Read the model definition and answer for the solid it produces. Units are mm, in the model's axes. Face numbers are marked on the shaded views. A direction names the side the tool comes from. Round coordinates to 2 decimals unless told otherwise and drop trailing zeros. Loops run counter-clockwise (first coordinate to the right, second up) from the corner with the lowest first, then second, coordinate; pieces in that order, holes last. Notation, with made-up numbers: M 27.5,43 L 48.5,43 A8 ccw 48.5,51 Z; hole C 25.5,-6.75 d4. An arc over 180 degrees is marked long. Write each question's results on one line, items separated by ' | '.
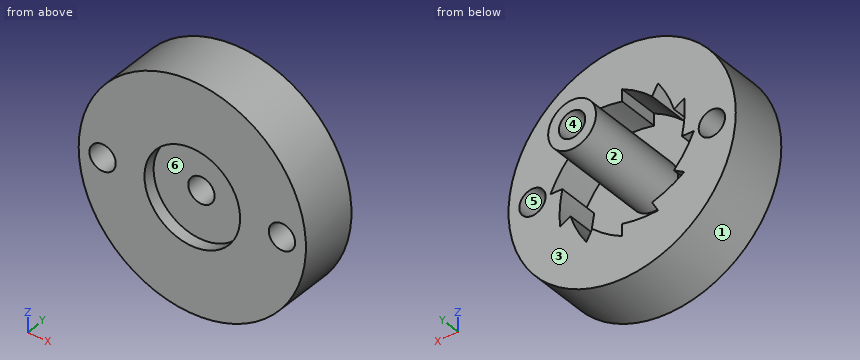
from build123d import *

# Parameters (mm, degrees)
SIDE_PROFILE_RATCHETING_PULLEY_MASTERMOD_W = 7.5
SIDE_PROFILE_RATCHETING_PULLEY_MASTERMOD_H = 5
RATCHETING_START                           = 1.5
RATCHETING_PULLEY_MASTERMODEL_OUTLINE_R    = 6
RATCHETING_PULLEY_MASTERMODEL_OUTLINE_R_2  = 2
RATCHETING_PULLEY_MASTERMODEL_DEPTH        = 3.5
M2_CLEARANCE_HOLE2_D                       = 2.2
BOSS_EXTRUDE2_DEPTH                        = 5
BOSS_EXTRUDE1_START                        = 10.5
BOTTOM_PULLEY_RATCHETING_PULLEY_MASTERMO_R = 2
BOSS_EXTRUDE1_DEPTH                        = 10.5
M2_CLEARANCE_HOLE3_D                       = 2.2
BOTTOM_PULLEY_RATCHETING_PULLEY_MAST_2_R   = 4
CUT_EXTRUDE3_DEPTH                         = 1


# Read off the part's stored shape, not the designer's step: ratcheting pulley mastermodel
with BuildPart() as part:
    # side profile-ratcheting pulley mastermod → Revolve1 (revolve)
    with BuildSketch(Plane.XY, mode=Mode.PRIVATE) as revolve1_sk:
        with Locations((-5.75, 2.5)):
            Rectangle(SIDE_PROFILE_RATCHETING_PULLEY_MASTERMOD_W, SIDE_PROFILE_RATCHETING_PULLEY_MASTERMOD_H)
        with Locations((5.75, 2.5)):
            Rectangle(SIDE_PROFILE_RATCHETING_PULLEY_MASTERMOD_W, SIDE_PROFILE_RATCHETING_PULLEY_MASTERMOD_H)
    revolve(revolve1_sk.sketch.rotate(Axis((0, 0, 0), (0, 1, 0)), 180), axis=Axis((0, 0, 0), (0, 1, 0)))

    # ratcheting pulley mastermodel outline → ratcheting pulley mastermodel (cut)
    with BuildSketch(Plane(origin=(0, 0, 0), x_dir=(1, 0, 0), z_dir=(0, 1, 0)).offset(RATCHETING_START)):
        Circle(RATCHETING_PULLEY_MASTERMODEL_OUTLINE_R)
        Circle(RATCHETING_PULLEY_MASTERMODEL_OUTLINE_R_2, mode=Mode.SUBTRACT)
    extrude(amount=RATCHETING_PULLEY_MASTERMODEL_DEPTH, mode=Mode.SUBTRACT)

    # M2 Clearance Hole2 (through all)
    with Locations(Plane(origin=(0, 0, 0), x_dir=(-1, 0, 0), z_dir=(0, -1, 0))):
        with Locations((-7.5, 0), (7.5, 0)):
            Hole(M2_CLEARANCE_HOLE2_D / 2)

    # ratchet profile-ratcheting pulley master → Boss-Extrude2 (add)
    with BuildSketch(Plane(origin=(0, 0, 0), x_dir=(1, 0, 0), z_dir=(0, 1, 0))):
        with BuildLine():
            ThreePointArc((-3, 5.196152423), (-1.492401284, 5.214292716), (0, 5))
            Line((0, 5), (0, 6))
            ThreePointArc((0, 6), (-1.552914271, 5.795554958), (-3, 5.196152423))
        make_face()
        with BuildLine():
            ThreePointArc((0, 6), (1.314688934, 5.261910597), (2.5, 4.330127019))
            Line((2.5, 4.330127019), (3, 5.196152423))
            ThreePointArc((3, 5.196152423), (1.552914271, 5.795554958), (0, 6))
        make_face()
        with BuildLine():
            ThreePointArc((3, 5.196152423), (3.769509313, 3.899603782), (4.330127019, 2.5))
            Line((4.330127019, 2.5), (5.196152423, 3))
            ThreePointArc((5.196152423, 3), (4.242640687, 4.242640687), (3, 5.196152423))
        make_face()
        with BuildLine():
            ThreePointArc((5.196152423, 3), (5.214292716, 1.492401284), (5, 0))
            Line((5, 0), (6, 0))
            ThreePointArc((6, 0), (5.795554958, 1.552914271), (5.196152423, 3))
        make_face()
        with BuildLine():
            ThreePointArc((6, 0), (5.261910597, -1.314688934), (4.330127019, -2.5))
            Line((4.330127019, -2.5), (5.196152423, -3))
            ThreePointArc((5.196152423, -3), (5.795554958, -1.552914271), (6, 0))
        make_face()
        with BuildLine():
            ThreePointArc((5.196152423, -3), (3.899603782, -3.769509313), (2.5, -4.330127019))
            Line((2.5, -4.330127019), (3, -5.196152423))
            ThreePointArc((3, -5.196152423), (4.242640687, -4.242640687), (5.196152423, -3))
        make_face()
        with BuildLine():
            ThreePointArc((3, -5.196152423), (1.492401284, -5.214292716), (0, -5))
            Line((0, -5), (0, -6))
            ThreePointArc((0, -6), (1.552914271, -5.795554958), (3, -5.196152423))
        make_face()
        with BuildLine():
            ThreePointArc((0, -6), (-1.314688934, -5.261910597), (-2.5, -4.330127019))
            Line((-2.5, -4.330127019), (-3, -5.196152423))
            ThreePointArc((-3, -5.196152423), (-1.552914271, -5.795554958), (0, -6))
        make_face()
        with BuildLine():
            ThreePointArc((-3, -5.196152423), (-3.769509313, -3.899603782), (-4.330127019, -2.5))
            Line((-4.330127019, -2.5), (-5.196152423, -3))
            ThreePointArc((-5.196152423, -3), (-4.242640687, -4.242640687), (-3, -5.196152423))
        make_face()
        with BuildLine():
            ThreePointArc((-5.196152423, -3), (-5.214292716, -1.492401284), (-5, 0))
            Line((-5, 0), (-6, 0))
            ThreePointArc((-6, 0), (-5.795554958, -1.552914271), (-5.196152423, -3))
        make_face()
        with BuildLine():
            ThreePointArc((-6, 0), (-5.261910597, 1.314688934), (-4.330127019, 2.5))
            Line((-4.330127019, 2.5), (-5.196152423, 3))
            ThreePointArc((-5.196152423, 3), (-5.795554958, 1.552914271), (-6, 0))
        make_face()
        with BuildLine():
            ThreePointArc((-5.196152423, 3), (-3.899603782, 3.769509313), (-2.5, 4.330127019))
            Line((-2.5, 4.330127019), (-3, 5.196152423))
            ThreePointArc((-3, 5.196152423), (-4.242640687, 4.242640687), (-5.196152423, 3))
        make_face()
    extrude(amount=BOSS_EXTRUDE2_DEPTH)

    # bottom pulley-ratcheting pulley mastermo → Boss-Extrude1 (add)
    with BuildSketch(Plane(origin=(0, 0, 0), x_dir=(1, 0, 0), z_dir=(0, 1, 0)).offset(BOSS_EXTRUDE1_START)):
        with Locations(Location((0, 0, 0), (0, 0, 270))):
            Circle(BOTTOM_PULLEY_RATCHETING_PULLEY_MASTERMO_R)
    extrude(amount=-BOSS_EXTRUDE1_DEPTH)

    # M2 Clearance Hole3 (through all)
    with Locations(Plane(origin=(0, 10.5, 0), x_dir=(1, 0, 0), z_dir=(0, 1, 0))):
        with Locations((0, 0)):
            Hole(M2_CLEARANCE_HOLE3_D / 2)

    # bottom pulley-ratcheting pulley mast 2 → Cut-Extrude3 (cut)
    with BuildSketch(Plane(origin=(0, 0, 0), x_dir=(1, 0, 0), z_dir=(0, 1, 0))):
        with Locations(Location((0, 0, 0), (0, 0, 270))):
            Circle(BOTTOM_PULLEY_RATCHETING_PULLEY_MAST_2_R)
    extrude(amount=CUT_EXTRUDE3_DEPTH, mode=Mode.SUBTRACT)


solid = part.part
Item 1: The part is cut by section D-D (x = -7.5). Determine the outline of the cut face in (y, z).
Outcome:
outline: M 0,-5.83 L 5,-5.83 L 5,-1.1 L 0,-1.1 Z; M 0,1.1 L 5,1.1 L 5,5.83 L 0,5.83 Z
Item 2: For the marked faces 5 and 6, determine the directions among +Z, -Z, +X, -X, +Y, -Y from which every point of the face is accessible in a straight line to the end or side of a thin tool.
Outcome:
face 5: +Y, -Y | face 6: -Y
Item 3: The part is cut by section C-C (z = -5.75). Determine the outline of the cut face in (x, y), plus the area to 3 significant figures.
Outcome:
outline: M -7.56,0 L 7.56,0 L 7.56,5 L 0.5,5 L 0.5,1.5 L 0,1.5 L 0,5 L -7.56,5 Z | area: 73.9 mm2
Item 4: The mould has two halves that part along X. Classify the marked faces 1, 2, 3 and 4: pulls with the +X half, pulls with the -X half, needs draft (parallel to the pull), parting line crosses it, or undercut.
Outcome:
face 1: parting line crosses it | face 2: undercut | face 3: needs draft | face 4: undercut
Item 5: The part is cut by section A-A (x = 0.75). Determine the outline of the cut face in (y, z), plus the area to 3 significant figures.
Outcome:
outline: M 0,-9.47 L 5,-9.47 L 5,-5.61 L 1.5,-5.61 L 1.5,-1.85 L 10.5,-1.85 L 10.5,-0.8 L 1,-0.8 L 1,-3.93 L 0,-3.93 Z; M 0,3.93 L 1,3.93 L 1,0.8 L 10.5,0.8 L 10.5,1.85 L 1.5,1.85 L 1.5,5.14 L 5,5.14 L 5,9.47 L 0,9.47 Z | area: 67.3 mm2
Item 6: Flat-ended cylindrical pins translate along their axes: pin 1 (1.5 mm diameter, centred on x = -6.5, y = 3.5, fed in from -Z); pin 2 (1.3 mm diameter, centred on x = 7.5, z = 0, fed in from -Y); pin 3 (2 mm diameter, centred on x = -2, y = 1.5, fed in from +Z); pin 4 (0.5 mm diameter, centred on y = 3.5, z = -5.5, fed in from +X). Find the tip coordinate at first contact, or state that the pin passes through.
Outcome:
pin 1: stops at z = -7.56 | pin 2: passes through | pin 3: stops at z = 9.45 | pin 4: stops at x = 7.92
Item 7: The part is cut by section B-B (y = 9.75). Determine the outline of the cut face in (x, z).
Outcome:
outline: C 0,0 d4; hole C 0,0 d2.2
Item 8: Straight lines are drawn through the part: line 1 (Z direction, x = -4.75, y = 4.5); line 2 (X direction, y = 2, z = 1.5); line 3 (Y direction, x = 5.75, z = -5.75). For each, find the intervals that lie inside material, in ascending order.
Outcome:
line 1: z = -8.23 to -3.3, -2.74 to -2.01, 2.74 to 8.23 | line 2: x = -9.38 to -5.21, -1.32 to 1.32, 5.14 to 9.38 | line 3: y = 0 to 5
